Input: part model. Units: mm. Frame: model coordinates. A direction names the side the tool comes from. Round coordinates to 2 decimals unless told otherwise and drop trailing zeros. Loops run counter-clockwise (first coordinate to the right, second up) from the corner with the lowest first, then second, coordinate; pieces in that order, holes last.
(1) Cut plane A-A, the plane x = 368.3. Output: boundary loops of the cut face in (y, z), and give its area (3 significant figures).
(2) Line query: line 1 (Y direction, x = 323.5, z = 1); line 2 (Y direction, x = 368.3, z = 3.75); line 3 (X direction, y = 56.5, z = 5). Output: solid intervals per line, ascending.
(3) Cut plane B-B, the plane y = 19.05. Output: boundary loops of the cut face in (x, z), and give its area (3 significant figures).
(4) Cut plane C-C, the plane z = 3.25. Give the number of separate pieces and of enclosed holes in the cut face, and give its area (3 significant figures).
(5) Access query for faces 1 (the face through (114, 8.89, 3)), 2 (the face through (0, 39, 3)). Directions: +Z, -Z, +X, -X, +Y, -Y. A direction counts if a zero-diameter tool reaches every point of the face in a straight line with its end or side. Return the directions, or none.
from build123d import *

# Parameters (mm, degrees)
F0_W     = 12.7
F0_H     = 2.54
F0_R     = 3.3782
F1_DEPTH = 6.35


with BuildPart() as f1:
    # F0 (on Top) → F1 (new body)
    with BuildSketch(Plane.XY):
        Polygon((0, 69.85), (0, 0), (406.4, 0), (406.4, 76.2), (0, 76.2), align=None)
        with Locations((12.7, 7.62)):
            Rectangle(F0_W, F0_H, mode=Mode.SUBTRACT)
        with Locations((63.5, 7.62)):
            Rectangle(F0_W, F0_H, mode=Mode.SUBTRACT)
        with Locations((88.9, 7.62)):
            Rectangle(F0_W, F0_H, mode=Mode.SUBTRACT)
        with Locations((114.3, 7.62)):
            Rectangle(F0_W, F0_H, mode=Mode.SUBTRACT)
        with Locations((139.7, 7.62)):
            Rectangle(F0_W, F0_H, mode=Mode.SUBTRACT)
        with Locations((165.1, 7.62)):
            Rectangle(F0_W, F0_H, mode=Mode.SUBTRACT)
        with Locations((190.5, 7.62)):
            Rectangle(F0_W, F0_H, mode=Mode.SUBTRACT)
        with Locations((38.1, 19.05)):
            Circle(F0_R, mode=Mode.SUBTRACT)
        with Locations((215.9, 7.62)):
            Rectangle(F0_W, F0_H, mode=Mode.SUBTRACT)
        with Locations((241.3, 7.62)):
            Rectangle(F0_W, F0_H, mode=Mode.SUBTRACT)
        with Locations((266.7, 7.62)):
            Rectangle(F0_W, F0_H, mode=Mode.SUBTRACT)
        with Locations((292.1, 7.62)):
            Rectangle(F0_W, F0_H, mode=Mode.SUBTRACT)
        with Locations((317.5, 7.62)):
            Rectangle(F0_W, F0_H, mode=Mode.SUBTRACT)
        with Locations((342.9, 7.62)):
            Rectangle(F0_W, F0_H, mode=Mode.SUBTRACT)
        with Locations((393.7, 7.62)):
            Rectangle(F0_W, F0_H, mode=Mode.SUBTRACT)
        with Locations((368.3, 19.05)):
            Circle(F0_R, mode=Mode.SUBTRACT)
        with Locations((38.1, 57.15)):
            Circle(F0_R, mode=Mode.SUBTRACT)
        with Locations((12.7, 68.58)):
            Rectangle(F0_W, F0_H, mode=Mode.SUBTRACT)
        with Locations((63.5, 68.58)):
            Rectangle(F0_W, F0_H, mode=Mode.SUBTRACT)
        with Locations((88.9, 68.58)):
            Rectangle(F0_W, F0_H, mode=Mode.SUBTRACT)
        with Locations((114.3, 68.58)):
            Rectangle(F0_W, F0_H, mode=Mode.SUBTRACT)
        with Locations((139.7, 68.58)):
            Rectangle(F0_W, F0_H, mode=Mode.SUBTRACT)
        with Locations((165.1, 68.58)):
            Rectangle(F0_W, F0_H, mode=Mode.SUBTRACT)
        with Locations((190.5, 68.58)):
            Rectangle(F0_W, F0_H, mode=Mode.SUBTRACT)
        with Locations((215.9, 68.58)):
            Rectangle(F0_W, F0_H, mode=Mode.SUBTRACT)
        with Locations((241.3, 68.58)):
            Rectangle(F0_W, F0_H, mode=Mode.SUBTRACT)
        with Locations((266.7, 68.58)):
            Rectangle(F0_W, F0_H, mode=Mode.SUBTRACT)
        with Locations((292.1, 68.58)):
            Rectangle(F0_W, F0_H, mode=Mode.SUBTRACT)
        with Locations((368.3, 57.15)):
            Circle(F0_R, mode=Mode.SUBTRACT)
        with Locations((317.5, 68.58)):
            Rectangle(F0_W, F0_H, mode=Mode.SUBTRACT)
        with Locations((342.9, 68.58)):
            Rectangle(F0_W, F0_H, mode=Mode.SUBTRACT)
        with Locations((393.7, 68.58)):
            Rectangle(F0_W, F0_H, mode=Mode.SUBTRACT)
    extrude(amount=F1_DEPTH)


solid = f1.part
Reported:
1. outline: (0, 0) - (15.67, 0) - (15.67, 6.35) - (0, 6.35) - close; (22.43, 0) - (53.77, 0) - (53.77, 6.35) - (22.43, 6.35) - close; (60.53, 0) - (76.2, 0) - (76.2, 6.35) - (60.53, 6.35) - close
1. area: 398 mm2
2. line 1: y = 0 to 6.35, 8.89 to 67.31, 69.85 to 76.2
2. line 2: y = 0 to 15.67, 22.43 to 53.77, 60.53 to 76.2
2. line 3: x = 0 to 34.78, 41.42 to 364.98, 371.62 to 406.4
3. outline: (0, 0) - (34.72, 0) - (34.72, 6.35) - (0, 6.35) - close; (41.48, 0) - (364.92, 0) - (364.92, 6.35) - (41.48, 6.35) - close; (371.68, 0) - (406.4, 0) - (406.4, 6.35) - (371.68, 6.35) - close
3. area: 2,490 mm2
4. separate pieces: 1
4. enclosed holes: 32
4. area: 29,900 mm2
5. face 1: +Z, -Z
5. face 2: +Z, -Z, -X, +Y, -Y
